Read the model definition and answer for the solid it produces. Units are mm, in the model's axes. A direction names the side the tool comes from. Give positions to 0.01 mm unless a question says otherwise; leave off trailing zeros. Loops run counter-clockwise (first coordinate to the right, second up) from the corner with the lowest first, then second, coordinate; pieces in that order, holes last. Notation, with made-up numbers: (-9.5, 15.5) - (12.5, 15.5) arc R36 ccw to (12.5, 51.5) - close; hole circle Ø9 at (50.5, -34). An arc over 180 degrees is marked (long way). Use a Markdown table: item, result. Add a question column.
Item 1: A cutting plane is placed at C-C (z = -73.5). Determine the outline of the cut face in (x, y).
Item 2: Consider probe 1 along X at (y, z) = (143, -39); probe 2 along X at (y, z) = (204, -200.5); probe 3 along Y at (x, z) = (28, -241.5). Determine where each line is inside the solid, lowest interval first. Write a range as [from, to].
Item 3: Which of the six approach directions +Z, -Z, +X, -X, +Y, -Y give full straight-line access (tool end or side, diameter ignored) to faces 1 (the face through (43, 112.5, -45)), 2 (the face through (42.02, 169.54, -144.93)), 3 (the face through (35, 155, -130))?
Item 4: Each of these flat-tipped pins is pushed along its axis until it touches: P1, Ø19.5, axis at x = 37, y = 167.5, coming from the -Z side; P2, Ø11, axis at x = 42, z = -203, coming from the -Y side; P3, Ø19.5, axis at x = 40, y = 141.5, coming from the +Z side. Where does it stop, or does it pass through?
Item 5: For a pull along Z with two mould halves and no side action, classify faces 4 (the face through (35, 155, -100)), 5 (the face through (5, 114, 0)), 6 (the face through (35, 155, -250)) as +Z half, -Z half, draft (parallel to the pull), parting line (faces both ways), or undercut.
Item 6: A cutting plane is placed at B-B (y = 91.5). Determine the outline of the cut face in (x, z).
Item 7: A cutting plane is placed at A-A (x = 26). Give the number of separate pieces and of enclosed holes in the cut face, plus the area to 3 significant figures.
from build123d import *

# Parameters (mm, degrees)
SKETCH2_W           = 270
SKETCH2_H           = 225
BOSS_EXTRUDE1_DEPTH = 10
BOSS_EXTRUDE4_DEPTH = 270
SKETCH5_W           = 64.951905284
SKETCH5_H           = 10
CUT_EXTRUDE1_DEPTH  = 302.95039014


with BuildPart() as part:
    # Sketch2 → Boss-Extrude1 (new body)
    with BuildSketch(Plane(origin=(0, 0, 0), x_dir=(0, 0, -1), z_dir=(1, 0, 0))):
        with Locations((135, 112.5)):
            Rectangle(SKETCH2_W, SKETCH2_H)
    extrude(amount=BOSS_EXTRUDE1_DEPTH)

    # Sketch4 → Boss-Extrude4 (add)
    with BuildSketch(Plane.XY):
        Polygon((10, 225), (74.951905284, 112.5), (10, 112.5), align=None)
    extrude(amount=-BOSS_EXTRUDE4_DEPTH)

    # Sketch5 → Cut-Extrude1 (cut, through all)
    with BuildSketch(Plane.XZ.offset(-112.5)):
        with Locations((42.475952642, -265)):
            Rectangle(SKETCH5_W, SKETCH5_H)
        with Locations((42.475952642, -255)):
            Rectangle(SKETCH5_W, SKETCH5_H)
        with Locations((42.475952642, -235)):
            Rectangle(SKETCH5_W, SKETCH5_H)
        with Locations((42.475952642, -215)):
            Rectangle(SKETCH5_W, SKETCH5_H)
        with Locations((42.475952642, -195)):
            Rectangle(SKETCH5_W, SKETCH5_H)
        with Locations((42.475952642, -175)):
            Rectangle(SKETCH5_W, SKETCH5_H)
        with Locations((42.475952642, -155)):
            Rectangle(SKETCH5_W, SKETCH5_H)
        with Locations((42.475952642, -135)):
            Rectangle(SKETCH5_W, SKETCH5_H)
        with Locations((42.475952642, -115)):
            Rectangle(SKETCH5_W, SKETCH5_H)
        with Locations((42.475952642, -95)):
            Rectangle(SKETCH5_W, SKETCH5_H)
        with Locations((42.475952642, -75)):
            Rectangle(SKETCH5_W, SKETCH5_H)
        with Locations((42.475952642, -55)):
            Rectangle(SKETCH5_W, SKETCH5_H)
        with Locations((42.475952642, -35)):
            Rectangle(SKETCH5_W, SKETCH5_H)
        with Locations((42.475952642, -15)):
            Rectangle(SKETCH5_W, SKETCH5_H)
        with Locations((42.475952642, -5)):
            Rectangle(SKETCH5_W, SKETCH5_H)
    extrude(amount=-CUT_EXTRUDE1_DEPTH, mode=Mode.SUBTRACT)


solid = part.part
Geometry says:
| question | item | result |
|---|---|---|
| 1 | outline | (0, 0) - (10, 0) - (10, 225) - (0, 225) - close |
| 2 | probe 1 | [0, 10] |
| 2 | probe 2 | [0, 22.12] |
| 2 | probe 3 | [112.5, 193.82] |
| 3 | face 1 | +Z, -Z, +X, -Y |
| 3 | face 2 | +Z, -Z, +X, +Y |
| 3 | face 3 | +X, +Y, -Y |
| 4 | P1 | z = -250 |
| 4 | P2 | y = 112.5 |
| 4 | P3 | z = -20 |
| 5 | face 4 | undercut |
| 5 | face 5 | +Z half |
| 5 | face 6 | -Z half |
| 6 | outline | (0, -270) - (10, -270) - (10, 0) - (0, 0) - close |
| 7 | separate pieces | 12 |
| 7 | enclosed holes | 0 |
| 7 | area | 10,200 mm² |
